Could you check a few things on this model? Use its own coordinates, in mm. A direction names the side the tool comes from. Give positions to 0.01 mm unless a question says otherwise; leave off trailing zeros. Write each loop counter-clockwise with the first axis right and the second up, starting at its lowest first coordinate (ties: lowest second). Pieces come first, ordered by that corner, then holes. Notation, with made-up numbers: M 49,35 L 92,35 A21 ccw 92,69 Z; hole C -1,20.5 d11. An arc over 180 degrees is marked long. Use one line per item in the form item = value.
from build123d import *

# Parameters (mm, degrees)
SM_BASE_FLANGE_1_DEPTH = 2
OTHER_START            = -4.5
OTHER_1_DEPTH          = 20
OTHER_1_2_OUTLINE_W    = 2
OTHER_1_2_OUTLINE_H    = 24
OTHER_1_2_DEPTH        = 20
OTHER_START_2          = 5.5
OTHER_1_3_OUTLINE_W    = 2
OTHER_1_3_OUTLINE_H    = 15
OTHER_1_3_OUTLINE_H_2  = 9
OTHER_1_3_DEPTH        = 10
OTHER_START_3          = 4.5
OTHER_1_4_OUTLINE_W    = 2
OTHER_1_4_OUTLINE_H    = 15
OTHER_1_4_DEPTH        = 1
OTHER_2_DEPTH          = 20
OTHER_2_2_DEPTH        = 9
OTHER_2_3_DEPTH        = 11
OTHER_2_4_DEPTH        = 9
SKETCH_4_R             = 1.6
CUT_EXTRUDE_1_DEPTH    = 10
SKETCH_6_R             = 1.6
CUT_EXTRUDE_2_DEPTH    = 10
CUT_EXTRUDE_3_DEPTH    = 67
SKETCH_10_R            = 1.6
CUT_EXTRUDE_4_DEPTH    = 67
FILLET_1_R             = 3
FILLET_2_R             = 2


# Read off the part's stored shape, not the designer's step: 绘制的折弯1, 绘制的折弯2
# Sheet-metal steps are written as plain solids
with BuildPart() as part:
    # Sketch 1 → 基体-法兰1 (new body)
    with BuildSketch(Plane(origin=(0, 0, 0), x_dir=(1, 0, 0), z_dir=(0, 1, 0))):
        Polygon((-16, -15.5), (16, -15.5), (73, -15.5), (73, -4.5), (58, -4.5), (58, 4.5), (34, 4.5), (34, -5.5), (25, -5.5), (25, 4.5), (16, 4.5), (16, 15.5), (-16, 15.5), align=None)
    extrude(amount=-SM_BASE_FLANGE_1_DEPTH)

    # Other 1 outline → Other 1 (cut)
    with BuildSketch(Plane.XY.offset(OTHER_START)):
        with BuildLine():
            ThreePointArc((22.107630798, 0), (21.011254481, -1.449489743), (19.279203673, -2))
            Line((19.279203673, -2), (73, -2))
            Line((73, -2), (73, 0))
            Line((73, 0), (22.107630798, 0))
        make_face()
    extrude(amount=OTHER_1_DEPTH, mode=Mode.SUBTRACT)

    # Other 1 2 outline → Other 1 2 (add)
    with BuildSketch(Plane.XY.offset(OTHER_START)):
        with Locations((21.279203673, 24.579203673)):
            Rectangle(OTHER_1_2_OUTLINE_W, OTHER_1_2_OUTLINE_H)
        with BuildLine():
            Line((22.279203673, 1), (22.279203673, 3.579203673))
            Line((22.279203673, 3.579203673), (20.279203673, 3.579203673))
            Line((20.279203673, 3.579203673), (20.279203673, 1))
            ThreePointArc((20.279203673, 1), (19.986310454, 0.292893219), (19.279203673, 0))
            Line((19.279203673, 0), (22.107630798, 0))
            ThreePointArc((22.107630798, 0), (22.235999352, 0.492694064), (22.279203673, 1))
        make_face()
    extrude(amount=OTHER_1_2_DEPTH)

    # Other 1 3 outline → Other 1 3 (add)
    with BuildSketch(Plane.XY.offset(OTHER_START_2)):
        with Locations((21.279203673, 44.079203673)):
            Rectangle(OTHER_1_3_OUTLINE_W, OTHER_1_3_OUTLINE_H)
        with Locations((21.279203673, 8.079203673)):
            Rectangle(OTHER_1_3_OUTLINE_W, OTHER_1_3_OUTLINE_H_2)
    extrude(amount=OTHER_1_3_DEPTH)

    # Other 1 4 outline → Other 1 4 (add)
    with BuildSketch(Plane.XY.offset(OTHER_START_3)):
        with Locations((21.279203673, 44.079203673)):
            Rectangle(OTHER_1_4_OUTLINE_W, OTHER_1_4_OUTLINE_H)
    extrude(amount=OTHER_1_4_DEPTH)

    # Other 2 outline → Other 2 (cut)
    with BuildSketch(Plane.XY.offset(OTHER_START)):
        with BuildLine():
            ThreePointArc((20.279203673, 37.836834471), (21.728693416, 36.740458154), (22.279203673, 35.008407346))
            Line((22.279203673, 35.008407346), (22.279203673, 51.579203673))
            Line((22.279203673, 51.579203673), (20.279203673, 51.579203673))
            Line((20.279203673, 51.579203673), (20.279203673, 37.836834471))
        make_face()
    extrude(amount=OTHER_2_DEPTH, mode=Mode.SUBTRACT)

    # Other 2 2 outline → Other 2 2 (cut)
    with BuildSketch(Plane.XY.offset(OTHER_START)):
        Polygon((20.279203673, 36.008407347), (20.85, 36.579203673), (20.279203673, 36.579203673), align=None)
    extrude(amount=OTHER_2_2_DEPTH, mode=Mode.SUBTRACT)

    # Other 2 3 outline → Other 2 3 (add)
    with BuildSketch(Plane.XY.offset(OTHER_START_3)):
        with BuildLine():
            ThreePointArc((20.279203673, 37.836834471), (19.786509609, 37.965203025), (19.279203673, 38.008407346))
            Line((19.279203673, 38.008407346), (5.85, 38.008407346))
            Line((5.85, 38.008407346), (5.85, 36.008407346))
            Line((5.85, 36.008407346), (19.279203673, 36.008407346))
            ThreePointArc((19.279203673, 36.008407346), (19.986310455, 35.715514128), (20.279203673, 35.008407346))
            Line((20.279203673, 35.008407346), (20.279203673, 37.836834471))
        make_face()
    extrude(amount=OTHER_2_3_DEPTH)

    # Other 2 4 outline → Other 2 4 (add)
    with BuildSketch(Plane.XY.offset(OTHER_START)):
        with BuildLine():
            ThreePointArc((21.835098605, 36.579203673), (21.633955222, 36.867209419), (21.400524017, 37.12972769))
            Line((21.400524017, 37.12972769), (20.85, 36.579203673))
            Line((20.85, 36.579203673), (21.835098605, 36.579203673))
        make_face()
        with BuildLine():
            Line((20.279203673, 35.008407346), (20.279203673, 36.008407347))
            Line((20.279203673, 36.008407347), (19.986310454, 35.715514128))
            ThreePointArc((19.986310454, 35.715514128), (20.203083206, 35.391090779), (20.279203673, 35.008407346))
        make_face()
    extrude(amount=OTHER_2_4_DEPTH)

    # 草图4 → 切除-拉伸1 (cut)
    with BuildSketch(Plane(origin=(0, -2, 0), x_dir=(-1, 0, 0), z_dir=(0, -1, 0))):
        with Locations(Location((-12.5, 12.5, 0), (0, 0, 90))):
            Circle(SKETCH_4_R)
        with Locations(Location((12.5, 12.5, 0), (0, 0, 90))):
            Circle(SKETCH_4_R)
    extrude(amount=-CUT_EXTRUDE_1_DEPTH, mode=Mode.SUBTRACT)

    # 草图6 → 切除-拉伸2 (cut)
    with BuildSketch(Plane(origin=(0, -2, 0), x_dir=(-1, 0, 0), z_dir=(0, -1, 0))):
        with Locations(Location((12.8, -12.3, 0), (0, 0, 90))):
            Circle(SKETCH_6_R)
        with Locations(Location((4.5, -12.3, 0), (0, 0, 90))):
            Circle(SKETCH_6_R)
    extrude(amount=-CUT_EXTRUDE_2_DEPTH, mode=Mode.SUBTRACT)

    # 草图8 → 切除-拉伸3 (cut)
    with BuildSketch(Plane(origin=(0, 38.008407346, 0), x_dir=(1, 0, 0), z_dir=(0, 1, 0))):
        with BuildLine():
            Line((7.25, -10), (8.85, -10))
            Line((8.85, -10), (10.45, -10))
            ThreePointArc((10.45, -10), (8.85, -8.4), (7.25, -10))
        make_face()
        with BuildLine():
            Line((10.45, -10), (8.85, -10))
            Line((8.85, -10), (7.25, -10))
            ThreePointArc((7.25, -10), (8.85, -11.6), (10.45, -10))
        make_face()
        with BuildLine():
            ThreePointArc((17.5, -10), (15.85, -8.35), (14.2, -10))
            Line((14.2, -10), (15.85, -10))
            Line((15.85, -10), (17.5, -10))
        make_face()
        with BuildLine():
            Line((15.85, -10), (14.2, -10))
            ThreePointArc((14.2, -10), (15.85, -11.65), (17.5, -10))
            Line((17.5, -10), (15.85, -10))
        make_face()
    extrude(amount=-CUT_EXTRUDE_3_DEPTH, mode=Mode.SUBTRACT)

    # 草图10 → 切除-拉伸4 (cut)
    with BuildSketch(Plane.ZY.offset(-20.279203673)):
        with Locations(Location((10.3, 8.408407346, 0), (0, 0, 270))):
            Circle(SKETCH_10_R)
        with Locations(Location((10.3, 17.408407346, 0), (0, 0, 270))):
            Circle(SKETCH_10_R)
        with Locations(Location((10.3, 26.408407346, 0), (0, 0, 270))):
            Circle(SKETCH_10_R)
        with Locations(Location((0.3, 26.408407346, 0), (0, 0, 270))):
            Circle(SKETCH_10_R)
    extrude(amount=-CUT_EXTRUDE_4_DEPTH, mode=Mode.SUBTRACT)

    # 圆角1
    fillet_1_edges = [part.edges().sort_by_distance(p)[0] for p in [
        (21.279203673, 12.579203673, -4.5),
        (21.279203673, 3.579203673, -4.5),
        (16, -1, -15.5),
        (5.85, 37.008407346, 4.5),
        (5.85, 37.008407346, 15.5),
        (-16, -1, 15.5),
        (-16, -1, -15.5),
    ]]
    fillet(fillet_1_edges, radius=FILLET_1_R)

    # 圆角2
    fillet_2_edges = [part.edges().sort_by_distance(p)[0] for p in [
        (21.279203673, 3.579203673, 5.5),
        (21.279203673, 12.579203673, 5.5),
    ]]
    fillet(fillet_2_edges, radius=FILLET_2_R)


solid = part.part
1) For pin 1 Ø0.6 at (x, z) = (21, 2) entering from -Y; pin 2 Ø2 at (x, z) = (15.85, 10) entering from +Y (3 decimals); pin 3 Ø2 at (x, z) = (6, -3) entering from +Y; pin 4 Ø1 at (x, z) = (21, 1.5) entering from +Y, each with a flat end and sliding along its axis, tell me the tip position at first contact or that it passes through.
Checked values:
pin_1 = -1.64
pin_2 = through
pin_3 = 0
pin_4 = 37.13
2) I want a section at A-A, the plane x = -10. Please give me the cut outline in (y, z), plus the area to 3 significant figures.
Checked values:
outline = M -2,-15.5 L 0,-15.5 L 0,15.5 L -2,15.5 Z
area = 62.0 mm2
3) If I drill on L1, parallel to Y at x = 18, z = 12.5; L2, parallel to Z at x = 15.85, y = 37.35; L3, parallel to Y at x = -12.5, z = 1.5, over which ranges is the centre line in solid material (lowest first)?
Checked values:
L1 = -2 to 0, 36.01 to 38.01
L2 = 4.5 to 8.35, 11.65 to 15.5
L3 = -2 to 0
4) For faces 1 (the flat face through (15, 37, 4.5)), 2 (the cylindrical face through (21.29, 12.01, 4.9)), 3 (the cylindrical face through (19.994, 0.301, 5.36)), 4 (the flat face through (5.85, 37, 10)), which set-ups out of +Z, -Z, +X, -X, +Y, -Y let a thin tool reach every point of the face, with its end or its side?
Checked values:
face_1 = -Z, -X, +Y
face_2 = -Z, +X, -X
face_3 = +Z, -Z, -X
face_4 = +Z, -Z, -X, +Y
5) I want a section at B-B, the plane y = 4.5. Please give me the cut outline in (x, z), plus the area to 3 significant figures.
Checked values:
outline = M 20.28,5.18 L 22.28,5.18 L 22.28,15.5 L 20.28,15.5 Z
area = 20.6 mm2
6) Thinking about a two-plate mould opening in Z: for faces 5 (the flat face through (13, 38.008, 10)), 6 (the cylindrical face through (8.11, -0.99, 8.58)), 7 (the cylindrical face through (-15.14, -1.01, -14.6)), which applies, released by +Z, released by -Z, zero draft, split by the parting line, or undercut?
Checked values:
face_5 = zero draft
face_6 = undercut
face_7 = released by -Z
